Verification items for the finished model (mm, model axes). Give positions to 0.01 mm unless a question says otherwise; leave off trailing zeros. Loops run counter-clockwise (first coordinate to the right, second up) from the corner with the lowest first, then second, coordinate; pieces in that order, holes last. Notation, with made-up numbers: (-3.75, -5.5) - (2.25, -5.5) arc R17 ccw to (2.25, 15.5) - close; hole circle Ø2 at (-30, 78). An arc over 180 degrees is marked (long way). One line per item, written item: value. Start each with the question number.
1. Gauge pin test, flat end, axial feed: pin 1 (1 mm diameter, centred on y = 1.5, z = 5.5, fed in from -X). Record the tip position at first contact, or that the pin passes through.
2. Sectioned sample at A-A (y = 0). Record the cut outline in (x, z) (3 decimals).
3. Sectioned sample at B-B (z = 1). Record the cut outline in (x, y) (3 decimals).
4. Sectioned sample at D-D (y = 9.5). Record the cut outline in (x, z), plus the area to 3 significant figures.
5. Sectioned sample at C-C (x = -27). Record the cut outline in (y, z), plus the area to 3 significant figures.
6. Scan lines: L1, parallel to Y at x = 25.4, z = 3.5; L2, parallel to Y at x = -25.4, z = 4.25 (3 decimals); L3, parallel to X at y = 12, z = 3. Record each from-to range of solid material in increasing order. Write a range as [from, to].
7. Mould release check, pull along Y, two halves, no side actions. Record for faces 1 (the cylindrical face through (-41.906, -0.363, 3.131)), 2 (the cylindrical face through (-16.697, 0.036, 3.131)), 3 (the flat face through (0, -16.51, 3)): pulls with the +Y half, pulls with the -Y half, needs draft (parallel to the pull), parting line crosses it, or undercut.
from build123d import *

# Parameters (mm, degrees)
SKETCH1_R           = 2.159
SKETCH1_R_2         = 3.175
BOSS_EXTRUDE1_DEPTH = 6.35
SKETCH2_R           = 7.759647624
SKETCH2_R_2         = 3.81
BOSS_EXTRUDE2_DEPTH = 1.27
SKETCH3_R           = 0.829532788
SKETCH3_R_2         = 0.792789718
CUT_EXTRUDE1_DEPTH  = 17.272


with BuildPart() as part:
    # Sketch1 → Boss-Extrude1 (new body)
    with BuildSketch(Plane.XY):
        with BuildLine():
            Line((-25.4, 16.51), (25.4, 16.51))
            ThreePointArc((25.4, 16.51), (41.91, 0), (25.4, -16.51))
            Line((25.4, -16.51), (-25.4, -16.51))
            ThreePointArc((-25.4, -16.51), (-41.91, 0), (-25.4, 16.51))
        make_face()
        with Locations((25.4, 0)):
            Circle(SKETCH1_R, mode=Mode.SUBTRACT)
        with Locations((-25.4, 0)):
            Circle(SKETCH1_R_2, mode=Mode.SUBTRACT)
    extrude(amount=BOSS_EXTRUDE1_DEPTH)

    # Sketch2 → Boss-Extrude2 (add)
    with BuildSketch(Plane.XY.offset(6.35)):
        with Locations((25.4, 0)):
            Circle(SKETCH2_R)
        with Locations((25.4, 0)):
            Circle(SKETCH2_R_2, mode=Mode.SUBTRACT)
    extrude(amount=-BOSS_EXTRUDE2_DEPTH)

    # Sketch3 → Cut-Extrude1 (cut)
    with BuildSketch(Plane(origin=(0, 0, 0), x_dir=(-1, 0, 0), z_dir=(0, 0, -1))):
        with Locations((17.526, 0)):
            Circle(SKETCH3_R)
        with Locations((33.274, 0)):
            Circle(SKETCH3_R_2)
    extrude(amount=-CUT_EXTRUDE1_DEPTH, mode=Mode.SUBTRACT)


solid = part.part
Results are:
1. pin 1: stops at x = -41.88
2. outline: (-41.91, 0) - (-34.067, 0) - (-34.067, 6.35) - (-41.91, 6.35) - close; (-32.481, 0) - (-28.575, 0) - (-28.575, 6.35) - (-32.481, 6.35) - close; (-22.225, 0) - (-18.356, 0) - (-18.356, 6.35) - (-22.225, 6.35) - close; (-16.696, 0) - (23.241, 0) - (23.241, 6.35) - (-16.696, 6.35) - close; (27.559, 0) - (41.91, 0) - (41.91, 6.35) - (27.559, 6.35) - close
3. outline: (-25.4, -16.51) - (25.4, -16.51) arc R16.51 ccw to (25.4, 16.51) - (-25.4, 16.51) arc R16.51 ccw to start; hole circle Ø1.586 at (-33.274, 0); hole circle Ø6.35 at (-25.4, 0); hole circle Ø1.659 at (-17.526, 0); hole circle Ø4.318 at (25.4, 0)
4. outline: (-38.9, 0) - (38.9, 0) - (38.9, 6.35) - (-38.9, 6.35) - close
4. area: 494 mm^2
5. outline: (-16.43, 0) - (-2.74, 0) - (-2.74, 6.35) - (-16.43, 6.35) - close; (2.74, 0) - (16.43, 0) - (16.43, 6.35) - (2.74, 6.35) - close
5. area: 174 mm^2
6. L1: y = [-16.51, -2.16], [2.16, 16.51]
6. L2: y = [-16.51, -3.175], [3.175, 16.51]
6. L3: x = [-36.74, 36.74]
7. face 1: parting line crosses it
7. face 2: undercut
7. face 3: pulls with the -Y half
